Input: part model. Units: mm. Frame: model coordinates. Face numbers are marked on the shaded views. A direction names the side the tool comes from. Give positions to 0.01 mm unless a question says otherwise; leave off trailing zeros. Loops run counter-clockwise (first coordinate to the right, second up) from the corner with the lowest first, then second, coordinate; pieces in that order, holes last. Notation, with made-up numbers: M -34.5,88 L -22.5,88 A15 ccw -22.5,105 Z; hole C -27,12.25 d7. An arc over 180 degrees is marked long. Answer as a JSON object with one key per item and string values. Group by question number.
1) Ray query, L1, parallel to X at y = -39.5, z = -0.25; L2, parallel to Y at x = -17, z = -0.5; L3, parallel to Y at x = 0, z = 10.4. Return the intervals inside material, ascending.
2) Section query D-D on z = 10. Return loops of the section in (x, y), plus the area to 3 significant figures.
3) Section query A-A on y = -93. Return loops of the section in (x, z), plus the area to 3 significant figures.
4) Section query C-C on x = 0. Count the separate pieces of the cut face and the enclosed holes in it, plus the area to 3 significant figures.
5) Section query B-B on x = 24.5. Return loops of the section in (y, z), plus the area to 3 significant figures.
6) First-contact query: P1, Ø1.6, axis at y = 26, z = -0.5, coming from the -X side; P2, Ø4, axis at x = -12.5, z = 2.5, coming from the -Y side; P3, Ø18.5, axis at x = -9, y = -43.5, coming from the +Z side. Flat tips, straight axial feed; report the tip coordinate or a pass-through.
7) Access query for the marked faces 1 and 2. Directions: +Z, -Z, +X, -X, +Y, -Y. A direction counts if a zero-diameter tool reaches every point of the face in a straight line with its end or side. Return the directions, or none.
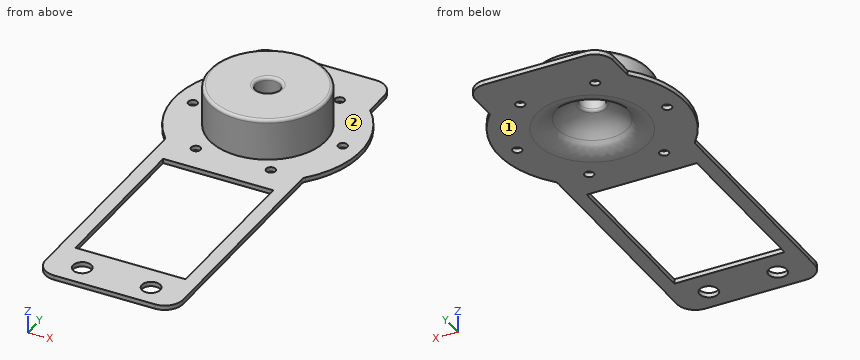
from build123d import *

# Parameters (mm, degrees)
CYLINDER010_R     = 19
CYLINDER010_DEPTH = 15
CYLINDER011_R     = 4
CYLINDER011_DEPTH = 18
SKETCH006_R       = 19
SKETCH006_R_2     = 3
SKETCH006_R_3     = 1.5
SKETCH006_W       = 36
SKETCH006_H       = 53.986387
PAD002_DEPTH      = 1.5
FILLET007_R       = 1
FILLET008_R       = 8


with BuildPart() as part:
    # Cylinder010 → Cylinder010 (join)
    with BuildSketch(Plane.XY):
        Circle(CYLINDER010_R)
    extrude(amount=CYLINDER010_DEPTH)

    # Sphere001 → Sphere001 (revolve, cut)
    with BuildSketch(Plane(origin=(0, 0, -5), x_dir=(1, 0, 0), z_dir=(0, -1, 0))):
        with BuildLine():
            ThreePointArc((0, -14.2), (14.2, 0), (0, 14.2))
            Line((0, 14.2), (0, -14.2))
        make_face()
    revolve(axis=Axis((0, 0, -5), (0, 0, 1)), mode=Mode.SUBTRACT)

    # Cylinder011 → Cylinder011 (cut)
    with BuildSketch(Plane.XY.offset(-2)):
        Circle(CYLINDER011_R)
    extrude(amount=CYLINDER011_DEPTH, mode=Mode.SUBTRACT)

    # Sketch006 → Pad002 (join)
    with BuildSketch(Plane.XY):
        with BuildLine():
            ThreePointArc((-22.5, 20.591260282), (-30.4977615184, 0.369516399), (-22.9922965207, -20.0400673827))
            ThreePointArc((-22.5, -21.3541501425), (-22.6271147127, -20.652515071), (-22.9922965208, -20.0400673827))
            Line((-22.5, -21.3541501425), (-22.5, -30.5))
            Line((-22.5, -30.5), (-22.5, -94.4863863704))
            ThreePointArc((-22.5, -94.4863863704), (-20.7426407961, -98.72902721), (-16.5000000467, -100.4863866319))
            Line((-16.5000000467, -100.4863866319), (16.5, -100.4863866319))
            ThreePointArc((16.5, -100.4863866319), (20.7426406871, -98.729027319), (22.5, -94.4863866319))
            Line((22.5, -94.4863866319), (22.5, -30.5))
            Line((22.5, -21.3541565041), (22.5, -30.5))
            ThreePointArc((22.9923076923, -20.0400545654), (22.6271165793, -20.6525100886), (22.5, -21.3541565041))
            ThreePointArc((22.9923076923, -20.0400545654), (30.4977614154, 0.3695248997), (22.5, 20.591260282))
            Line((22.5, 29.5), (22.5, 20.591260282))
            ThreePointArc((22.5, 29.5), (20.7426406871, 33.7426406871), (16.5, 35.5))
            Line((-16.5, 35.5), (16.5, 35.5))
            ThreePointArc((-16.5, 35.5), (-20.7426406871, 33.7426406871), (-22.5, 29.5))
            Line((-22.5, 20.591260282), (-22.5, 29.5))
        make_face()
        Circle(SKETCH006_R, mode=Mode.SUBTRACT)
        with Locations((-11.25, -93)):
            Circle(SKETCH006_R_2, mode=Mode.SUBTRACT)
        with Locations((11.25, -93)):
            Circle(SKETCH006_R_2, mode=Mode.SUBTRACT)
        with Locations((-12.25, 21.217622)):
            Circle(SKETCH006_R_3, mode=Mode.SUBTRACT)
        with Locations((12.25, 21.217622)):
            Circle(SKETCH006_R_3, mode=Mode.SUBTRACT)
        with Locations((24.5, 0)):
            Circle(SKETCH006_R_3, mode=Mode.SUBTRACT)
        with Locations((-24.5, 0)):
            Circle(SKETCH006_R_3, mode=Mode.SUBTRACT)
        with Locations((-12.25, -21.217622)):
            Circle(SKETCH006_R_3, mode=Mode.SUBTRACT)
        with Locations((12.25, -21.217622)):
            Circle(SKETCH006_R_3, mode=Mode.SUBTRACT)
        with Locations((0, -57.4931935)):
            Rectangle(SKETCH006_W, SKETCH006_H, mode=Mode.SUBTRACT)
    extrude(amount=PAD002_DEPTH)

    # Fillet007
    fillet007_edges = [part.edges().sort_by_distance(p)[0] for p in [
        (-19, 0, 15),
        (-4, 0, 15),
        (-4, 0, 8.624977),
    ]]
    fillet(fillet007_edges, radius=FILLET007_R)

    # Fillet008
    fillet008_edges = [part.edges().sort_by_distance(p)[0] for p in [
        (-13.290598, 0, 0),
    ]]
    fillet(fillet008_edges, radius=FILLET008_R)


with BuildPart() as part_1:
    # Body003 placement: moved
    add(part.part.moved(Location((0, 0, -1.5))))


solid = part_1.part
Output:
{
 "1": {"L1": "x = -22.5 to -18, 18 to 22.5", "L2": "y = -100.47 to -84.49, -30.5 to 35.48", "L3": "y = -19 to -4, 4 to 19"},
 "2": {"outline": "C 0,0 d38; hole C 0,0 d8", "area": "1,080 mm^2"},
 "3": {"outline": "M -22.5,-1.5 L -14.25,-1.5 L -14.25,0 L -22.5,0 Z; M -8.25,-1.5 L 8.25,-1.5 L 8.25,0 L -8.25,0 Z; M 14.25,-1.5 L 22.5,-1.5 L 22.5,0 L 14.25,0 Z", "area": "49.5 mm^2"},
 "4": {"separate pieces": "3", "enclosed holes": "0", "area": "403 mm^2"},
 "5": {"outline": "M -18.17,-1.5 L -1.5,-1.5 L -1.5,0 L -18.17,0 Z; M 1.5,-1.5 L 18.17,-1.5 L 18.17,0 L 1.5,0 Z", "area": "50.0 mm^2"},
 "6": {"P1": "stops at x = -22.5", "P2": "stops at y = -15.84", "P3": "stops at z = 0"},
 "7": {"face 1": "-Z, +X, -X, +Y, -Y", "face 2": "+Z"}
}
